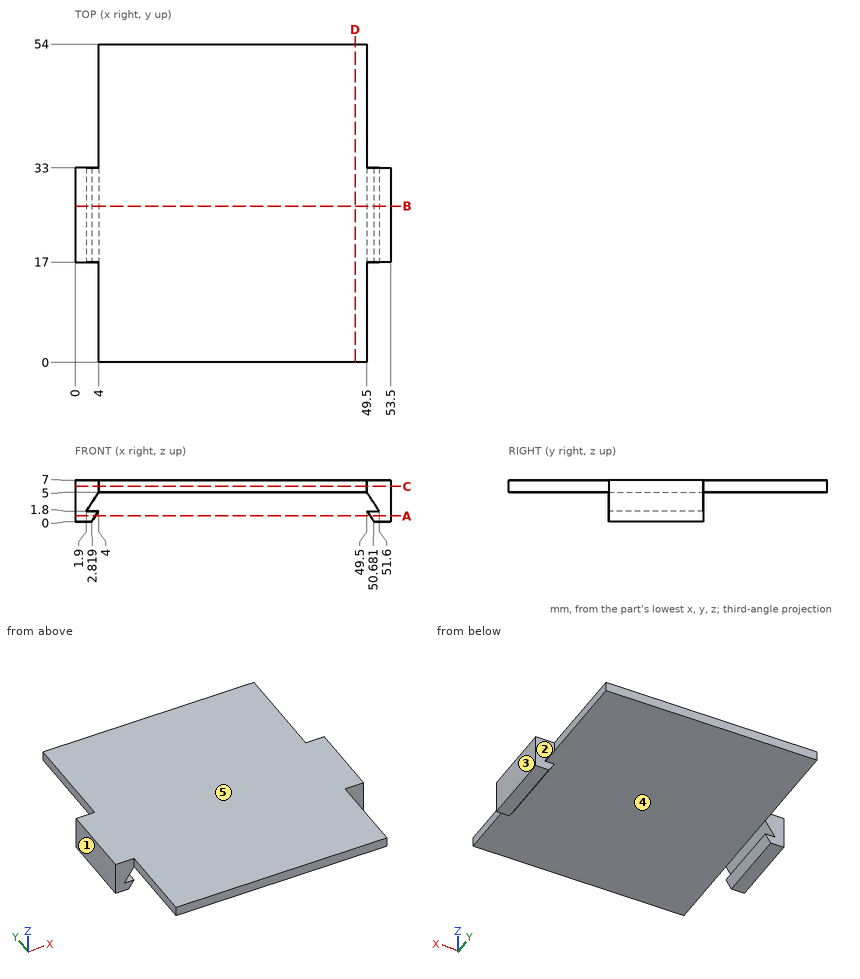
Geometry check sheet. Reference: drawing and pictorial views, mm from the part's lowest x, y, z. A direction names the side the tool comes from. Round coordinates to 2 decimals unless told otherwise and drop trailing zeros. Loops run counter-clockwise (first coordinate to the right, second up) from the corner with the lowest first, then second, coordinate; pieces in that order, holes last. Notation, with made-up numbers: (5.5, -23.75) - (53.5, -23.75) arc R25 cw to (53.5, -3.75) - close; hole circle Ø8 at (80, 84.25). An arc over 180 degrees is marked (long way). Answer in a Markdown table with one row per item. Add a question column.
Q1. Tool access check on the marked faces 1 and 2. Record the directions out of +Z, -Z, +X, -X, +Y, -Y that give a thin tool (end or side, any length) a straight path to the whole face; none if there is none.
Q2. Material ranges on line 1 (Z direction, x = 24, y = 39); line 2 (X direction, y = 34, z = 6.5); line 3 (X direction, y = 31.5, z = 1.5), recorded low to high.
Q3. Section check D-D on x = 47.5. Enter the section's corners in (y, z), plus the area to 3 significant figures.
Q4. Gauge pin test, flat ends, axial feed: pin 1 (2 mm diameter, centred on x = 51, z = 4, fed in from +Y); pin 2 (0.6 mm diameter, centred on y = 42.5, z = 6.5, fed in from +X); pin 3 (2 mm diameter, centred on y = 46.5, z = 5.5, fed in from -X). Record the tip position at first contact, or that the pin passes through.
Q5. Section check C-C on z = 6. Enter the section's corners in (x, y).
Q6. Section check B-B on y = 26.5. Enter the section's corners in (x, z), plus the area to 3 significant figures.
Q7. Section check A-A on z = 1. Enter the section's corners in (x, y) (1 decimal), plus the area to 3 significant figures.
Q8. Release check for a two-part mould opening along X. For the marked faces 3, 4 and 5 record: pulls with the +X half, pulls with the -X half, needs draft (parallel to the pull), parting line crosses it, or undercut.
Found:
| question | item | result |
|---|---|---|
| 1 | face 1 | +Z, -Z, -X, +Y, -Y |
| 1 | face 2 | +Z, -Z, +X, +Y |
| 2 | line 1 | z = 5 to 7 |
| 2 | line 2 | x = 4 to 49.5 |
| 2 | line 3 | x = 0 to 3.8, 49.7 to 53.5 |
| 3 | outline | (0, 5) - (54, 5) - (54, 7) - (0, 7) - close |
| 3 | area | 108 mm² |
| 4 | pin 1 | stops at y = 33 |
| 4 | pin 2 | stops at x = 49.5 |
| 4 | pin 3 | stops at x = 4 |
| 5 | outline | (0, 17) - (4, 17) - (4, 0) - (49.5, 0) - (49.5, 17) - (53.5, 17) - (53.5, 33) - (49.5, 33) - (49.5, 54) - (4, 54) - (4, 33) - (0, 33) - close |
| 6 | outline | (0, 0) - (2.82, 0) - (4, 1.8) - (1.9, 1.8) - (4, 5) - (49.5, 5) - (51.6, 1.8) - (49.5, 1.8) - (50.68, 0) - (53.5, 0) - (53.5, 7) - (0, 7) - close |
| 6 | area | 138 mm² |
| 7 | outline | (0, 17) - (3.5, 17) - (3.5, 33) - (0, 33) - close; (50, 17) - (53.5, 17) - (53.5, 33) - (50, 33) - close |
| 7 | area | 111 mm² |
| 8 | face 3 | pulls with the +X half |
| 8 | face 4 | undercut |
| 8 | face 5 | needs draft |
